Part model, mm, in its own coordinate system. A direction names the side the tool comes from. Round coordinates to 2 decimals unless told otherwise and drop trailing zeros. Loops run counter-clockwise (first coordinate to the right, second up) from the corner with the lowest first, then second, coordinate; pieces in that order, holes last.
(1) Tool access for faces 4 (the face through (74, 16, 3.35)), 5 (the face through (0.44, 54.29, 2.64)): list every direction of +Z, -Z, +X, -X, +Y, -Y with a clear straight run to the whole face (end or side of a thin tool).
(2) Flat gauge pins, fed straight in: pin 1 (2 mm diameter, centred on y = 22, z = 2.5, fed in from +X); pin 2 (1 mm diameter, centred on x = 60, z = 4, fed in from +Y). Where does each tip first touch, or does it go through?
(3) Cut at C-C on y = 27. List the corners of the cut face in (x, z).
(4) Mould opens along Y. For faces 1 (the face through (7, 7, 3)), 2 (the face through (43.957, 54.676, 0.764)), 3 (the face through (0, 27, 3)) say: +Y half, -Y half, draft (parallel to the pull), parting line (faces both ways), or undercut.
(5) Cut at B-B on x = 64. List the corners of the cut face in (y, z), then the cut area to 3 significant figures.
(6) Cut at A-A on y = 7. List the corners of the cut face in (x, z).
(7) Probe probe 1 along Y at (x, z) = (67.5, 2.45); probe 2 along Z at (x, y) = (63, 53); probe 3 along Z at (x, y) = (68.5, 8). List the from-to ranges inside material, lowest first.
(8) Cut at D-D on x = 14. List the corners of the cut face in (y, z), then the cut area to 3 significant figures.
from build123d import *

# Parameters (mm, degrees)
F0_W     = 86.7
F0_H     = 55.4
F1_DEPTH = 5.2
F2_R     = 2.54
F4_DEPTH = 25.4
F6_W     = 27
F6_H     = 1.5
F7_DEPTH = 25.4


with BuildPart() as f1:
    # F0 (on Top) → F1 (new body)
    with BuildSketch(Plane.XY):
        with Locations((43.35, 27.7)):
            Rectangle(F0_W, F0_H)
    extrude(amount=F1_DEPTH)

    # F2
    f2_edges = [f1.edges().sort_by_distance(p)[0] for p in [
        (43.35, 0, 5.2),
        (43.35, 0, 0),
        (43.35, 55.4, 5.2),
        (43.35, 55.4, 0),
        (86.7, 0, 2.6),
        (0, 0, 2.6),
        (0, 55.4, 2.6),
        (86.7, 55.4, 2.6),
    ]]
    fillet(f2_edges, radius=F2_R)

    # F3 (on face) → F4 (cut)
    with BuildSketch(Plane.XY.offset(5.2)):
        Polygon((9.5, 4.5), (4.5, 9.5), (4.5, 4.5), align=None)
    extrude(amount=-F4_DEPTH, mode=Mode.SUBTRACT)

    # F6 (on face) → F7 (cut)
    with BuildSketch(Plane.YZ.offset(86.7)):
        with Locations((16.5, 2.6)):
            Rectangle(F6_W, F6_H)
    extrude(amount=-F7_DEPTH, mode=Mode.SUBTRACT)


solid = f1.part
Final values:
1. face 4: +X
1. face 5: +Z, -Z, -X, +Y
2. pin 1: stops at x = 86.7
2. pin 2: stops at y = 55.26
3. outline: (0, 0) - (86.7, 0) - (86.7, 1.85) - (61.3, 1.85) - (61.3, 3.35) - (86.7, 3.35) - (86.7, 5.2) - (0, 5.2) - close
4. face 1: undercut
4. face 2: +Y half
4. face 3: draft
5. outline: (0, 2.54) arc R2.54 ccw to (2.54, 0) - (52.86, 0) arc R2.54 ccw to (55.4, 2.54) - (55.4, 2.66) arc R2.54 ccw to (52.86, 5.2) - (2.54, 5.2) arc R2.54 ccw to (0, 2.66) - close; hole (3, 1.85) - (30, 1.85) - (30, 3.35) - (3, 3.35) - close
5. area: 242 mm2
6. outline: (0, 0) - (4.5, 0) - (4.5, 5.2) - (0, 5.2) - close; (7, 0) - (86.7, 0) - (86.7, 1.85) - (61.3, 1.85) - (61.3, 3.35) - (86.7, 3.35) - (86.7, 5.2) - (7, 5.2) - close
7. probe 1: y = 0 to 3, 30 to 55.4
7. probe 2: z = 0 to 5.2
7. probe 3: z = 0 to 1.85, 3.35 to 5.2
8. outline: (0, 2.54) arc R2.54 ccw to (2.54, 0) - (52.86, 0) arc R2.54 ccw to (55.4, 2.54) - (55.4, 2.66) arc R2.54 ccw to (52.86, 5.2) - (2.54, 5.2) arc R2.54 ccw to (0, 2.66) - close
8. area: 283 mm2
